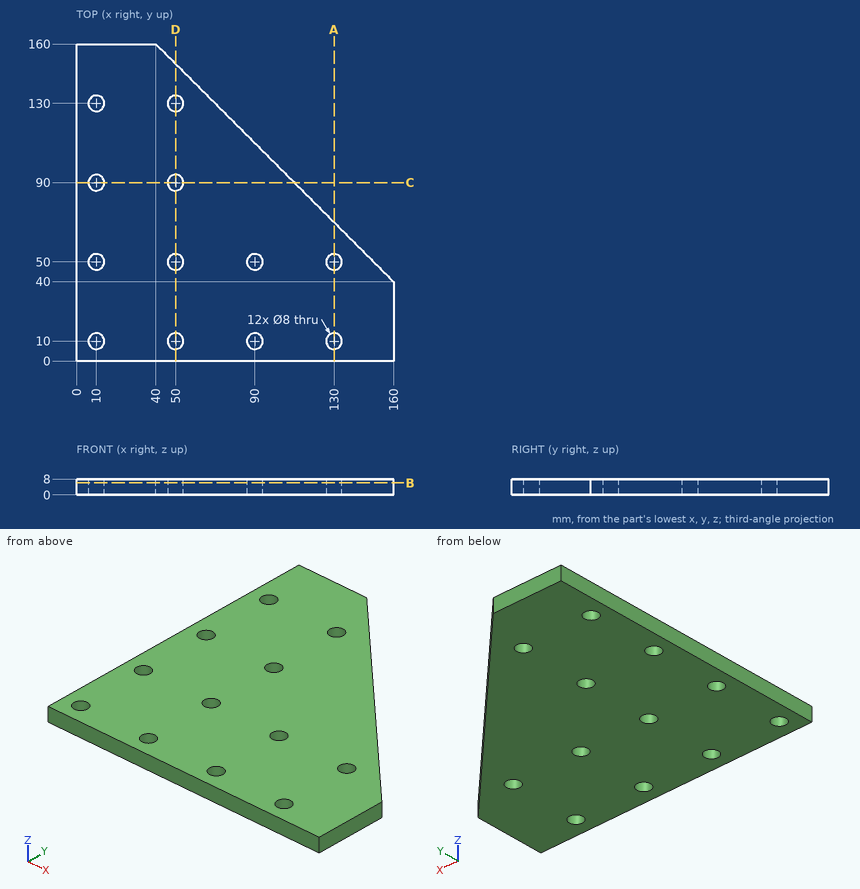
Study the drawing (mm; zero at the part's minimum x, y, z) and answer. Coordinates: 2 decimals unless noted, no trailing zeros. Write each loop counter-clockwise with the first axis right and the second up, starting at its lowest first coordinate (ties: lowest second). Pieces come first, ordered by that corner, then holes. Notation, with made-up numbers: (42.25, 24) - (61.25, 24) arc R30 cw to (61.25, 50) - close; hole circle Ø5 at (31.5, 88.25). An arc over 180 degrees is marked (long way). Answer as a JSON object with one key per item and string values. Group by question number.
1. A cutting plane is placed at A-A (x = 130). Determine the outline of the cut face in (y, z), plus the area to 3 significant figures.
2. A cutting plane is placed at D-D (x = 50). Determine the outline of the cut face in (y, z).
3. Each of these flat-tipped pins is pushed along its axis until it touches: P1, Ø3, axis at y = 50.5, z = 1, coming from the +X side; P2, Ø4, axis at x = 61.5, z = 1.5, coming from the +Y side. Where does it stop, or does it pass through?
4. A cutting plane is placed at B-B (z = 6). Give the number of separate pieces and of enclosed holes in the cut face, plus the area to 3 significant figures.
5. Consider L1, parallel to Y at x = 130, z = 5.25; L2, parallel to Y at x = 126.5, z = 3; L3, parallel to Y at x = 50, z = 6. Determine where each line is inside the solid, lowest interval first. Write a range as [from, to].
6. A cutting plane is placed at C-C (y = 90). Determine the outline of the cut face in (x, z), plus the area to 3 significant figures.
Worked out:
{
 "1": {"outline": "(0, 0) - (6, 0) - (6, 8) - (0, 8) - close; (14, 0) - (46, 0) - (46, 8) - (14, 8) - close; (54, 0) - (70, 0) - (70, 8) - (54, 8) - close", "area": "432 mm²"},
 "2": {"outline": "(0, 0) - (6, 0) - (6, 8) - (0, 8) - close; (14, 0) - (46, 0) - (46, 8) - (14, 8) - close; (54, 0) - (86, 0) - (86, 8) - (54, 8) - close; (94, 0) - (126, 0) - (126, 8) - (94, 8) - close; (134, 0) - (150, 0) - (150, 8) - (134, 8) - close"},
 "3": {"P1": "stops at x = 151", "P2": "stops at y = 140.5"},
 "4": {"separate pieces": "1", "enclosed holes": "12", "area": "17,800 mm²"},
 "5": {"L1": "y = [0, 6], [14, 46], [54, 70]", "L2": "y = [0, 8.06], [11.94, 48.06], [51.94, 73.5]", "L3": "y = [0, 6], [14, 46], [54, 86], [94, 126], [134, 150]"},
 "6": {"outline": "(0, 0) - (6, 0) - (6, 8) - (0, 8) - close; (14, 0) - (46, 0) - (46, 8) - (14, 8) - close; (54, 0) - (110, 0) - (110, 8) - (54, 8) - close", "area": "752 mm²"}
}
